from build123d import *

# Parameters (mm, degrees)
EXTRUDE_1_DEPTH     = 3
SKETCH_3_W          = 13.8
SKETCH_3_H          = 3
SKETCH_3_W_2        = 3
SKETCH_3_H_2        = 13.8
CUT_EXTRUDE_1_DEPTH = 10
EXTRUDE_START       = -3
EXTRUDE_2_DEPTH     = 3
FILLET_1_R          = 10
SKETCH_6_W          = 3
SKETCH_6_H          = 13.8
CUT_EXTRUDE_2_DEPTH = 10
SKETCH_7_R          = 1.5
CUT_EXTRUDE_3_DEPTH = 10
SKETCH_8_R          = 5
CUT_EXTRUDE_4_DEPTH = 10


with BuildPart() as part:
    # Эскиз2 → Бобышка-Вытянуть1 (new body)
    with BuildSketch(Plane(origin=(0, 0, 0), x_dir=(1, 0, 0), z_dir=(0, 1, 0))):
        with BuildLine():
            Line((50.901300831, -31.765666587), (63.52144012, -24.956238913))
            ThreePointArc((63.52144012, -24.956238913), (90, 0), (63.52144012, 24.956238913))
            Line((63.52144012, 24.956238913), (50.901300831, 31.765666587))
            ThreePointArc((50.901300831, 31.765666587), (-60, 0), (50.901300831, -31.765666587))
        make_face()
    extrude(amount=EXTRUDE_1_DEPTH)

    # Эскиз3 → Вырез-Вытянуть1 (cut)
    with BuildSketch(Plane(origin=(0, 3, 0), x_dir=(1, 0, 0), z_dir=(0, 1, 0))):
        with Locations((0, 53.956851754)):
            Rectangle(SKETCH_3_W, SKETCH_3_H)
        with Locations((0, -53.956851754)):
            Rectangle(SKETCH_3_W, SKETCH_3_H)
        with Locations((-53.60522772, 0)):
            Rectangle(SKETCH_3_W_2, SKETCH_3_H_2)
    extrude(amount=-CUT_EXTRUDE_1_DEPTH, mode=Mode.SUBTRACT)

    # Эскиз5 → Бобышка-Вытянуть2 (add)
    with BuildSketch(Plane(origin=(0, 3, 0), x_dir=(1, 0, 0), z_dir=(0, 1, 0)).offset(EXTRUDE_START)):
        with BuildLine():
            Line((111.52144012, 24.956238913), (66.47855988, 24.956238913))
            ThreePointArc((66.47855988, 24.956238913), (90, 0), (66.47855988, -24.956238913))
            Line((66.47855988, -24.956238913), (111.52144012, -24.956238913))
            Line((111.52144012, -24.956238913), (111.52144012, 24.956238913))
        make_face()
    extrude(amount=EXTRUDE_2_DEPTH)

    # Скругление1
    fillet_1_edges = [part.edges().sort_by_distance(p)[0] for p in [
        (111.52144012, 1.5, 24.956238913),
        (111.52144012, 1.5, -24.956238913),
    ]]
    fillet(fillet_1_edges, radius=FILLET_1_R)

    # Эскиз6 → Вырез-Вытянуть2 (cut)
    with BuildSketch(Plane(origin=(0, 3, 0), x_dir=(1, 0, 0), z_dir=(0, 1, 0))):
        with Locations((106.52144012, -0.043761087)):
            Rectangle(SKETCH_6_W, SKETCH_6_H)
    extrude(amount=-CUT_EXTRUDE_2_DEPTH, mode=Mode.SUBTRACT)

    # Эскиз7 → Вырез-Вытянуть3 (cut)
    with BuildSketch(Plane(origin=(0, 3, 0), x_dir=(1, 0, 0), z_dir=(0, 1, 0))):
        with Locations(Location((3, 0, 0), (0, 0, 270))):
            Circle(SKETCH_7_R)
    extrude(amount=-CUT_EXTRUDE_3_DEPTH, mode=Mode.SUBTRACT)

    # Эскиз8 → Вырез-Вытянуть4 (cut)
    with BuildSketch(Plane(origin=(0, 3, 0), x_dir=(1, 0, 0), z_dir=(0, 1, 0))):
        with Locations(Location((63.40144012, -0.703761087, 0), (0, 0, 270))):
            Circle(SKETCH_8_R)
    extrude(amount=-CUT_EXTRUDE_4_DEPTH, mode=Mode.SUBTRACT)


solid = part.part
Build history of the part. All positions in model axes, mm. Coordinates: 2 decimals unless noted, no trailing zeros. Order: outer loops, then holes, each group sorted by start corner. A loop starts at its lowest first (then second) coordinate and runs counter-clockwise, first axis right, second up. Notation, with made-up numbers: (6.25, 31.5) - (30.25, 31.5) arc R17 cw to (30.25, 50.5) - close; hole circle Ø6 at (62.5, 41.25). An arc over 180 degrees is marked (long way). Write each question's results on one line, items separated by ' | '. Start each with the question number.
Item 1: Mould opens along Z. For faces 1 (the face through (6, 0, -1)), 2 (the face through (68.36, 1.52, 0.05)), 3 (the face through (57.3, 1.479, -28.313)) say: released by +Z, released by -Z, zero draft, split by the parting line, or undercut.
Item 2: Band-saw the part on B-B on x = 71.5. Write the cut outline in (y, z).
Item 3: Band-saw the part on C-C on z = -48. Write the cut outline in (x, y).
Item 4: Wall check: probe 1 along X at (y, z) = (1.25, 1); probe 2 along X at (y, z) = (1, -1); probe 3 along Z at (x, y) = (3.5, 1.15). Give the ranges that are in metal, low to high. Write a range as [from, to].
Item 5: Band-saw the part on A-A on y = 1.6. Write the cut outline in (x, z), and give its area (3 significant figures).
Item 6: Flat gauge pins, fed straight in: pin 1 (0.9 mm diameter, centred on y = 1.5, z = 54.5, fed in from -X); pin 2 (0.9 mm diameter, centred on y = 1, z = -53.5, fed in from -X); pin 3 (0.9 mm diameter, centred on x = 2, y = 2, fed in from -Z). Where does each tip first touch, or does it go through?
Numbers:
1) face 1: zero draft | face 2: undercut | face 3: released by -Z
2) outline: (0, -24.96) - (3, -24.96) - (3, 24.96) - (0, 24.96) - close
3) outline: (-36, 0) - (36, 0) - (36, 3) - (-36, 3) - close
4) probe 1: [-59.99, -55.11], [-52.11, 1.88], [4.12, 58.41], [68.39, 105.02], [108.02, 111.52] | probe 2: [-59.99, -55.11], [-52.11, 1.88], [4.12, 58.7], [68.1, 105.02], [108.02, 111.52] | probe 3: [-59.9, -55.46], [-52.46, -1.41], [1.41, 52.46], [55.46, 59.9]
5) outline: (50.9, -31.77) - (63.52, -24.96) arc R25 ccw to (66.48, -24.96) - (101.52, -24.96) arc R10 ccw to (111.52, -14.96) - (111.52, 14.96) arc R10 ccw to (101.52, 24.96) - (66.48, 24.96) arc R25 ccw to (63.52, 24.96) - (50.9, 31.77) arc R60 ccw (long way) to start; hole (-55.11, -6.9) - (-52.11, -6.9) - (-52.11, 6.9) - (-55.11, 6.9) - close; hole (-6.9, -55.46) - (6.9, -55.46) - (6.9, -52.46) - (-6.9, -52.46) - close; hole (-6.9, 52.46) - (6.9, 52.46) - (6.9, 55.46) - (-6.9, 55.46) - close; hole circle Ø3 at (3, 0); hole circle Ø10 at (63.4, 0.7); hole (105.02, -6.86) - (108.02, -6.86) - (108.02, 6.94) - (105.02, 6.94) - close | area: 13,700 mm^2
6) pin 1: x = -26.05 | pin 2: x = -28.03 | pin 3: z = -59.98
